Geometry check sheet. Reference: the model listing, model coordinates, mm. A direction names the side the tool comes from. Round coordinates to 2 decimals unless told otherwise and drop trailing zeros. Write each loop counter-clockwise with the first axis right and the second up, starting at its lowest first coordinate (ties: lowest second). Pieces come first, ordered by that corner, then holes. Notation, with made-up numbers: (-9.5, 84.25) -> (42.5, 84.25) arc R35 ccw to (42.5, 117.25) -> close; hole circle Ø5 at (2, -24). An arc over 180 degrees is marked (long way). Return JSON: item names as keys, results as strings. Group by question number.
Autodesk Inventor part; units mm, degrees
ref_plane "YZ Plane" through (0, 0, 0) normal (1, 0, 0) x (0, 1, 0)
ref_plane "XZ Plane" through (0, 0, 0) normal (0, 1, 0) x (-1, 0, 0)
ref_plane "XY Plane" through (0, 0, 0) normal (0, 0, 1) x (1, 0, 0)
sketch "Sketch1" plane through (0, 0, 0) normal (0, 1, 0) x (-1, 0, 0)
  arc A0 (-2.75, 2.1651) -> (2.75, 2.1651) centre (0, 0) ccw
  line L0 (-1.9, 14.1) -> (-2.75, 2.1651)
  line L1 (1.8987, 14.0987) -> (2.75, 2.1651)
  arc A1 (1.8987, 14.0987) -> (-1.9, 14.1) centre (-0.0007, 14.05) ccw
  circle A2 centre (0, 0) radius 0.5
  arc A3 (-7.6535, 3.6978) -> (7.6533, 3.6982) centre (0, 0) ccw
  line L2 (-7.6535, 3.6978) -> (-6.8928, 14.3783)
  arc A4 (6.8916, 14.3762) -> (-6.8928, 14.3783) centre (-0.0007, 14.05) ccw
  line L3 (6.8916, 14.3762) -> (7.6533, 3.6982)
  point P0 (0, 15.95)
  dimension "d0" = 1
  dimension "d9" = 1.9
  dimension "d10" = 15.95
  dimension "d11" = 3.5
  dimension "d17" = 5
extrude "Extrusion1" add sketch "Sketch1" along normal blind 3.8 contours L2 A4 L3 A3
sketch "Sketch2" plane through (0, 3.8, 0) normal (0, 1, 0) x (1, 0, 0)
  arc A0 (2.75, -2.1651) -> (-2.75, -2.1651) centre (0, 0) ccw
  circle A1 centre (0, 0) radius 3.5
  arc A2 (-6.8916, -14.3762) -> (6.8928, -14.3783) centre (0.0007, -14.05) ccw
  line L0 (-7.6533, -3.6982) -> (-6.8916, -14.3762)
  arc A3 (7.6535, -3.6978) -> (-7.6533, -3.6982) centre (0, 0) ccw
  line L1 (6.8928, -14.3783) -> (7.6535, -3.6978)
  arc A4 (2.75, -2.1651) -> (-2.75, -2.1651) centre (0, 0) ccw
  point P0 (2.75, -2.1651)
  point P1 (-2.75, -2.1651)
extrude "Extrusion2" add sketch "Sketch2" along normal blind 5
sketch "Sketch3" plane through (0, 8.8, 0) normal (0, 1, 0) x (1, 0, 0)
  arc A0 (2.75, -2.1651) -> (-2.75, -2.1651) centre (0, 0) ccw
  circle A1 centre (0, 0) radius 5
  dimension "d22" = 10
extrude "Extrusion3" add sketch "Sketch3" along normal blind 8
sketch "Sketch4" plane through (0, 16.8, 0) normal (0, 1, 0) x (1, 0, 0)
  circle A0 centre (0, 0) radius 5
  line L0 (1, 3) -> (-1, 3)
  line L1 (-1, 3) -> (-1, 7)
  line L2 (-1, 7) -> (1, 7)
  line L3 (1, 7) -> (1, 3)
  line L4 (1, 3) -> (-1, 7) construction
  line L5 (-1, 3) -> (1, 7) construction
  point P0 (0, 5)
  point P1 (-1, 4.899)
  point P2 (1, 4.899)
  dimension "d25" = 10
  dimension "d26" = 2
  dimension "d27" = 4
  dimension "d28" = 1
extrude "Extrusion4" add sketch "Sketch4" along normal blind 25 contours A0 L1 L0 L3 picked at (-0.1517, 0.3403)
sketch "Sketch5" plane through (0, 3.8, 0) normal (0, -1, 0) x (1, 0, 0)
  circle A0 centre (0, 0) radius 3.5
  dimension "d31" = 7
extrude "Extrusion5" add sketch "Sketch5" against normal blind 5
properties part number "Servo_Shaft_V2"
1) Sectioned sample at C-C on x = 0. Enter the section's corners in (y, z).
2) Mould release check, pull along X, two halves, no side actions. Record for faces 1 (the face through (0, 29, -3)), 2 (the face through (-7.267, 4.338, 9.112)), 3 (the face through (0.04, 1.87, 15.95)), 4 (the face through (-0.241, 4.338, -8.497)): +X half, -X half, draft (parallel to the pull), parting line (faces both ways), or undercut.
3) Go/stop test with flat-tipped pins: P1, Ø0.9, axis at y = 27.5, z = -4, coming from the +X side; P2, Ø5, axis at x = -4, z = 17, coming from the +Y side; P3, Ø5, axis at y = 9.5, z = 15, coming from the +X side. Record where each tip stops, or that it passes through.
4) Sectioned sample at D-D on y = 32.5. Enter the section's corners in (x, z).
5) Material ranges on probe 1 along Z at (x, y) = (0, 2.75); probe 2 along X at (y, z) = (1.6, 0); probe 3 along Y at (x, z) = (4.5, 10.75), recorded low to high. Write a range as [from, to].
6) Tool access check on faces 5 (the face through (2.307, 25.069, -4.436)), 6 (the face through (7.28, 4.34, 8.96)), 7 (the face through (0, 16.8, -4)), 8 (the face through (2.32, 1.87, 8.22)), 9 (the face through (0, 41.8, 0)). Record the directions out of +Z, -Z, +X, -X, +Y, -Y that give a thin tool (end or side, any length) a straight path to the whole face; none if there is none.
7) Sectioned sample at B-B on z = 0. Enter the section's corners in (x, y).
8) Sectioned sample at A-A on y = 3. Enter the section's corners in (x, z).
Evaluation:
{
 "1": {"outline": "(0, -8.5) -> (8.8, -8.5) -> (8.8, -5) -> (16.8, -5) -> (16.8, -3) -> (41.8, -3) -> (41.8, 5) -> (8.8, 5) -> (8.8, 20.95) -> (0, 20.95) -> (0, 15.95) -> (3.8, 15.95) -> (3.8, -3.5) -> (0, -3.5) -> close"},
 "2": {"face 1": "undercut", "face 2": "-X half", "face 3": "undercut", "face 4": "parting line"},
 "3": {"P1": "stops at x = 3.52", "P2": "stops at y = 8.8", "P3": "stops at x = 7.02"},
 "4": {"outline": "(-1, -4.9) -> (-1, -3) -> (1, -3) -> (1, -4.9) arc R5 ccw (long way) to start"},
 "5": {"probe 1": "z = [-8.5, -3.5], [15.95, 20.95]", "probe 2": "x = [-8.5, -3.5], [3.5, 8.5]", "probe 3": "y = [0, 8.8]"},
 "6": {"face 5": "+Y", "face 6": "+Z, +X, +Y, -Y", "face 7": "-Z, +Y", "face 8": "-Y", "face 9": "+Z, -Z, +X, -X, +Y"},
 "7": {"outline": "(-8.5, 0) -> (-3.5, 0) -> (-3.5, 3.8) -> (3.5, 3.8) -> (3.5, 0) -> (8.5, 0) -> (8.5, 8.8) -> (5, 8.8) -> (5, 41.8) -> (-5, 41.8) -> (-5, 8.8) -> (-8.5, 8.8) -> close"},
 "8": {"outline": "(-7.65, 3.7) arc R8.5 ccw (long way) to (7.65, 3.7) -> (6.89, 14.38) arc R6.9 ccw to (-6.89, 14.38) -> close; hole (-2.75, 2.17) arc R3.5 ccw (long way) to (2.75, 2.17) -> (1.9, 14.1) arc R1.9 ccw to (-1.9, 14.1) -> close"}
}
